Here's how the part is built. I have some questions about the finished solid (model axes, mm). A direction names the side the tool comes from. Coordinates: 2 decimals unless noted, no trailing zeros. Write each loop counter-clockwise with the first axis right and the second up, starting at its lowest first coordinate (ties: lowest second). Pieces come first, ordered by that corner, then holes.
Item 1: If we section it at A-A (x = -42.5): Please give me the cut outline in (y, z) (1 decimal).
Item 2: We'd pull the mould along Z, two halves only. Please class faces 1 (the face through (-6, -12, -19.748)), 2 (the face through (-30, -11.307, -18)), 3 (the face through (-6.84, -14.89, -7.45)): +Z half, -Z half, draft (parallel to the pull), parting line (faces both ways), or undercut.
Item 3: If we section it at B-B (x = -3): Please give me the cut outline in (y, z) (1 decimal).
Item 4: If I drill on line 1 (Z direction, x = -41, y = -10.75); line 2 (Z direction, x = -37.5, y = -11.5); line 3 (X direction, y = -13.25, z = -16.5), over which ranges is the centre line in solid material (lowest first)?
Item 5: I'm going to push flat-ended pins straight in: pin 1 Ø0.7 at (x, y) = (-14, -12) entering from +Z; pin 2 Ø4.5 at (x, z) = (-2.5, -23) entering from +Y; pin 3 Ø3.5 at (x, y) = (-12.5, -15.5) entering from +Z. Where does each tip first touch, or does it pass through?
Item 6: For faces 4 (the face through (-20, -15, -16.891)), 5 (the face through (-33, -15, -29.845)), 6 (the face through (-46, -10.672, -8)), which set-ups out of +Z, -Z, +X, -X, +Y, -Y let a thin tool reach every point of the face, with its end or its side?
from build123d import *

# Parameters (mm, degrees)
SKETCH1_W           = 72.009
SKETCH1_H           = 6.985
BOSS_EXTRUDE1_DEPTH = 32.258
SKETCH2_W           = 13.335
SKETCH2_H           = 2.032
CUT_EXTRUDE1_DEPTH  = 75.682449945
SKETCH3_W           = 19.304
SKETCH3_H           = 2.921
CUT_EXTRUDE2_DEPTH  = 11.811
FILLET1_R           = 2.54
CUT_EXTRUDE3_DEPTH  = 75.682449945
SKETCH6_W           = 60.325
SKETCH6_H           = 2.413
CUT_EXTRUDE6_DEPTH  = 73.900474235
SKETCH11_W          = 18.161
SKETCH11_H          = 5.588
CUT_EXTRUDE7_DEPTH  = 3.429
SKETCH12_W          = 18.161
SKETCH12_H          = 3.175
CUT_EXTRUDE8_DEPTH  = 73.652144185
SKETCH13_W          = 30.314137033
SKETCH13_H          = 2.54
CUT_EXTRUDE9_DEPTH  = 10.0965
CUT_EXTRUDE10_DEPTH = 73.900474235
FILLET2_R           = 0.635
CUT_EXTRUDE11_DEPTH = 81.85576081
CUT_EXTRUDE12_DEPTH = 73.900474235
SKETCH18_R          = 0.758626194
SKETCH18_R_2        = 0.86735546
CUT_EXTRUDE13_DEPTH = 2.4765
SKETCH19_R          = 2.8575
CUT_EXTRUDE14_DEPTH = 73.733906314
CHAMFER1_SIZE       = 0.381
SKETCH20_R          = 1.651
CUT_EXTRUDE15_DEPTH = 73.900474235
CHAMFER2_SIZE       = 0.381
SKETCH21_R          = 2.159
CUT_EXTRUDE16_DEPTH = 73.900474235
SKETCH22_R          = 3.7465
CUT_EXTRUDE17_DEPTH = 4.572


with BuildPart() as part:
    # Sketch1 → Boss-Extrude1 (new body)
    with BuildSketch(Plane.XY):
        with Locations((-28.996348877, -14.164776435)):
            Rectangle(SKETCH1_W, SKETCH1_H)
    extrude(amount=-BOSS_EXTRUDE1_DEPTH)

    # Sketch2 → Cut-Extrude1 (cut, through all)
    with BuildSketch(Plane.XY):
        with Locations((-58.333348877, -16.641276435)):
            Rectangle(SKETCH2_W, SKETCH2_H)
    extrude(amount=-CUT_EXTRUDE1_DEPTH, mode=Mode.SUBTRACT)

    # Sketch3 → Cut-Extrude2 (cut)
    with BuildSketch(Plane.XY):
        with Locations((-5.183848877, -12.132776435)):
            Rectangle(SKETCH3_W, SKETCH3_H)
    extrude(amount=-CUT_EXTRUDE2_DEPTH, mode=Mode.SUBTRACT)

    # Fillet1
    fillet1_edges = [part.edges().sort_by_distance(p)[0] for p in [
        (-14.835848877, -13.593276435, -5.9055),
        (4.468151123, -13.593276435, -5.9055),
    ]]
    fillet(fillet1_edges, radius=FILLET1_R)

    # Sketch4 → Cut-Extrude3 (cut, through all)
    with BuildSketch(Plane.XY):
        Polygon((7.008151123, -17.657276435), (7.008151123, -15.498276435), (-1.754848877, -17.657276435), align=None)
    extrude(amount=-CUT_EXTRUDE3_DEPTH, mode=Mode.SUBTRACT)

    # Sketch6 → Cut-Extrude6 (cut, through all)
    with BuildSketch(Plane(origin=(0, -10.672276435, 0), x_dir=(1, 0, 0), z_dir=(0, 1, 0))):
        with Locations((-23.154348877, 31.0515)):
            Rectangle(SKETCH6_W, SKETCH6_H)
        with Locations((-23.154348877, 1.2065)):
            Rectangle(SKETCH6_W, SKETCH6_H)
    extrude(amount=-CUT_EXTRUDE6_DEPTH, mode=Mode.SUBTRACT)

    # Sketch11 → Cut-Extrude7 (cut)
    with BuildSketch(Plane(origin=(0, -10.672276435, 0), x_dir=(1, 0, 0), z_dir=(0, 1, 0))):
        with Locations((-39.537348877, 27.051)):
            Rectangle(SKETCH11_W, SKETCH11_H)
    extrude(amount=-CUT_EXTRUDE7_DEPTH, mode=Mode.SUBTRACT)

    # Sketch12 → Cut-Extrude8 (cut, through all)
    with BuildSketch(Plane(origin=(0, -14.101276435, 0), x_dir=(1, 0, 0), z_dir=(0, 1, 0))):
        with Locations((-39.537348877, 25.8445)):
            Rectangle(SKETCH12_W, SKETCH12_H)
    extrude(amount=-CUT_EXTRUDE8_DEPTH, mode=Mode.SUBTRACT)

    # Sketch13 → Cut-Extrude9 (cut)
    with BuildSketch(Plane(origin=(0, 0, -29.845), x_dir=(-1, 0, 0), z_dir=(0, 0, -1))):
        with Locations((5.139780361, -11.942276435)):
            Rectangle(SKETCH13_W, SKETCH13_H)
    extrude(amount=-CUT_EXTRUDE9_DEPTH, mode=Mode.SUBTRACT)

    # Sketch14 → Cut-Extrude10 (cut, through all)
    with BuildSketch(Plane(origin=(0, -10.672276435, 0), x_dir=(1, 0, 0), z_dir=(0, 1, 0))):
        Polygon((-20.296848877, 29.845), (7.008151123, 19.7485), (7.008151123, 29.845), align=None)
        Polygon((-20.296848877, 2.413), (7.008151123, 12.6365), (7.008151123, 2.413), align=None)
    extrude(amount=-CUT_EXTRUDE10_DEPTH, mode=Mode.SUBTRACT)

    # Fillet2
    fillet2_edges = [part.edges().sort_by_distance(p)[0] for p in [
        (-6.644348877, -13.212276435, -19.7485),
    ]]
    fillet(fillet2_edges, radius=FILLET2_R)

    # Sketch16 → Cut-Extrude11 (cut, through all)
    with BuildSketch(Plane.ZY.offset(65.000848877)):
        Polygon((-17.2085, -11.942276435), (-15.0495, -11.942276435), (-15.0495, -11.307276435), (-13.589, -11.307276435), (-13.589, -10.672276435), (-18.669, -10.672276435), (-18.669, -11.307276435), (-17.2085, -11.307276435), align=None)
    extrude(amount=-CUT_EXTRUDE11_DEPTH, mode=Mode.SUBTRACT)

    # Sketch17 → Cut-Extrude12 (cut, through all)
    with BuildSketch(Plane.XZ.offset(17.657276435)):
        Polygon((-31.002948877, -16.891), (-28.970948877, -16.891), (-28.958248877, -17.907), (-25.808648877, -17.907), (-25.808648877, -16.891), (-23.776648877, -16.891), (-23.763948877, -17.907), (-20.614348877, -17.907), (-20.614348877, -16.891), (-18.582348877, -16.891), (-18.569648877, -17.907), (-15.420048877, -17.907), (-15.420048877, -16.891), (-13.388048877, -16.891), (-13.375348877, -17.907), (-10.225748877, -17.907), (-10.225748877, -16.891), (-8.193748877, -16.891), (-8.168348877, -15.367), (-10.200348877, -15.367), (-10.200348877, -14.351), (-13.375348877, -14.351), (-13.362648877, -15.367), (-15.394648877, -15.367), (-15.394648877, -14.351), (-18.569648877, -14.351), (-18.556948877, -15.367), (-20.588948877, -15.367), (-20.588948877, -14.351), (-23.763948877, -14.351), (-23.751248877, -15.367), (-25.783248877, -15.367), (-25.783248877, -14.351), (-28.958248877, -14.351), (-28.945548877, -15.367), (-30.977548877, -15.367), (-30.977548877, -14.351), (-34.152548877, -14.351), (-34.139848877, -15.367), (-36.171848877, -15.367), (-36.171848877, -14.351), (-39.346848877, -14.351), (-39.346848877, -17.907), (-36.197248877, -17.907), (-36.197248877, -16.891), (-34.165248877, -16.891), (-34.152548877, -17.907), (-31.002948877, -17.907), align=None)
    extrude(amount=-CUT_EXTRUDE12_DEPTH, mode=Mode.SUBTRACT)

    # Sketch18 → Cut-Extrude13 (cut)
    with BuildSketch(Plane.XZ.offset(17.657276435)):
        with Locations((-8.829621314, -13.140704274)):
            Circle(SKETCH18_R)
        with Locations((-40.878405559, -14.788679648)):
            Circle(SKETCH18_R_2)
    extrude(amount=-CUT_EXTRUDE13_DEPTH, mode=Mode.SUBTRACT)

    # Sketch19 → Cut-Extrude14 (cut, through all)
    with BuildSketch(Plane.XZ.offset(15.625276435)):
        with Locations(Location((-59.158848877, -5.842, 0), (0, 0, 270))):
            Circle(SKETCH19_R)
        with Locations(Location((-59.158848877, -26.416, 0), (0, 0, 270))):
            Circle(SKETCH19_R)
    extrude(amount=-CUT_EXTRUDE14_DEPTH, mode=Mode.SUBTRACT)

    # Chamfer1
    chamfer1_edges = [part.edges().sort_by_distance(p)[0] for p in [
        (-59.158848877, -15.625276435, -2.9845),
        (-59.158848877, -15.625276435, -23.5585),
    ]]
    chamfer(chamfer1_edges, length=CHAMFER1_SIZE)

    # Sketch20 → Cut-Extrude15 (cut, through all)
    with BuildSketch(Plane.XZ.offset(17.657276435)):
        with Locations((-26.392848877, -8.255)):
            Circle(SKETCH20_R)
        with Locations((-26.392848877, -24.003)):
            Circle(SKETCH20_R)
    extrude(amount=-CUT_EXTRUDE15_DEPTH, mode=Mode.SUBTRACT)

    # Chamfer2
    chamfer2_edges = [part.edges().sort_by_distance(p)[0] for p in [
        (-28.043848877, -10.672276435, -8.255),
        (-28.043848877, -17.657276435, -8.255),
        (-28.043848877, -10.672276435, -24.003),
        (-28.043848877, -17.657276435, -24.003),
    ]]
    chamfer(chamfer2_edges, length=CHAMFER2_SIZE)

    # Sketch21 → Cut-Extrude16 (cut, through all)
    with BuildSketch(Plane.XZ.offset(17.657276435)):
        with Locations((-39.600848877, -9.468375809)):
            Circle(SKETCH21_R)
        with Locations((-18.645848877, -9.468375809)):
            Circle(SKETCH21_R)
    extrude(amount=-CUT_EXTRUDE16_DEPTH, mode=Mode.SUBTRACT)

    # Sketch22 → Cut-Extrude17 (cut)
    with BuildSketch(Plane(origin=(0, -10.672276435, 0), x_dir=(1, 0, 0), z_dir=(0, 1, 0))):
        with Locations(Location((-39.600848877, 9.468375809, 0), (0, 0, 270))):
            Circle(SKETCH22_R)
        with Locations(Location((-18.645848877, 9.468375809, 0), (0, 0, 270))):
            Circle(SKETCH22_R)
    extrude(amount=-CUT_EXTRUDE17_DEPTH, mode=Mode.SUBTRACT)


solid = part.part
Answer list:
1. outline: (-17.7, -29.8) - (-14.1, -29.8) - (-14.1, -27.4) - (-17.7, -27.4) - close; (-17.7, -24.3) - (-10.7, -24.3) - (-10.7, -18.7) - (-11.3, -18.7) - (-11.3, -17.2) - (-11.9, -17.2) - (-11.9, -15) - (-11.3, -15) - (-11.3, -13.6) - (-10.7, -13.6) - (-10.7, -11.8) - (-15.2, -11.8) - (-15.2, -7.1) - (-10.7, -7.1) - (-10.7, -2.4) - (-17.7, -2.4) - close
2. face 1: -Z half
2. face 2: undercut
2. face 3: +Z half
3. outline: (-17.7, -23.4) - (-13.2, -23.4) - (-13.2, -20.4) arc R0.6 cw to (-12.6, -19.7) - (-10.7, -19.7) - (-10.7, -18.7) - (-11.3, -18.7) - (-11.3, -17.2) - (-11.9, -17.2) - (-11.9, -15) - (-11.3, -15) - (-11.3, -13.6) - (-10.7, -13.6) - (-10.7, -11.8) - (-13.6, -11.8) - (-13.6, -8.9) - (-17.7, -8.9) - close
4. line 1: z = -24.26 to -18.67, -13.59 to -12.94, -5.99 to -2.41
4. line 2: z = -24.26 to -17.91, -14.35 to -12.57, -6.37 to -2.41
4. line 3: x = -65 to -39.35, -8.19 to 7.01
5. pin 1: stops at z = -11.81
5. pin 2: stops at y = -13.21
5. pin 3: stops at z = -4.68
6. face 4: +Y, -Y
6. face 5: -Z, +X, +Y, -Y
6. face 6: +Z, -Z, +X, -X, +Y
